from build123d import *


with BuildPart() as part:
    # Sketch1 → Revolve1 (revolve)
    with BuildSketch(Plane.XY, mode=Mode.PRIVATE) as revolve1_sk:
        with BuildLine():
            Line((137.291796068, 0), (141.645898034, 4.868033989))
            ThreePointArc((141.645898034, 4.868033989), (141.910434206, 6.565517768), (140.468847051, 7.5))
            Line((140.468847051, 7.5), (124, 7.5))
            Line((124, 7.5), (124, 5))
            Line((124, 5), (0, 5))
            Line((0, 5), (0, 0))
            Line((0, 0), (124, 0))
            Line((124, 0), (137.291796068, 0))
        make_face()
    revolve1 = revolve(revolve1_sk.sketch.rotate(Axis((0, 0, 0), (1, 0, 0)), 90), axis=Axis((0, 0, 0), (1, 0, 0)))

    # Mirror1: Revolve1 across plane
    add(revolve1.mirror(Plane.ZY))


solid = part.part
Design review of the part built by this model. Coordinates are the model's own, in mm. A direction names the side the tool comes from. Round coordinates to 2 decimals unless told otherwise and drop trailing zeros. Order: outer loops, then holes, each group sorted by start corner. A loop starts at its lowest first (then second) coordinate and runs counter-clockwise, first axis right, second up.
1) Clearance check with flat-ended pins moving along their axes: pin 1 Ø1 at (y, z) = (-1.5, 5.5) entering from +X; pin 2 Ø1.5 at (x, z) = (38.5, -4.5) entering from -Y; pin 3 Ø1 at (x, z) = (75.5, -3) entering from +Y; pin 4 Ø4.5 at (y, z) = (0, 1.5) entering from -X. State where each tip first meets the part, or that it passes through.
The answers:
pin 1: stops at x = 142.05
pin 2: stops at y = -3.31
pin 3: stops at y = 4.33
pin 4: stops at x = -140.65
2) Machinability: for faces 5 (the flat face through (-124, 5, 2)), 6 (the conical face through (-138.05, 0.83, -0.18)), which of the approach directions +Z, -Z, +X, -X, +Y, -Y give a long, thin tool a straight path to every point of the face, cutting with its end or side? Answer none if there is none.
The answers:
face 5: none
face 6: -X
3) Consider section A-A (x = 64). State the section outline as (y, z) points, plus the area to 3 significant figures.
The answers:
outline: circle Ø10 at (0, 0)
area: 78.5 mm2
4) Draft analysis for pull direction X (two halves, no side actions). For faces 1 (the flat face through (124, 5, 2)), 2 (the cylindrical face through (-132.119, -6.324, 4.032)), 3 (the conical face through (138.05, 0.83, -0.18)), 4 (the cylindrical face through (2, 0, -5)), state which applies: released by +X, released by -X, zero draft, split by the parting line, or undercut.
The answers:
face 1: undercut
face 2: zero draft
face 3: released by +X
face 4: undercut
5) For L1, parallel to Y at x = -111.5, z = -1.25; L2, parallel to X at y = -5, z = 2.75; L3, parallel to X at y = 1.5, z = -3.25, list the stretches that pass through material, from the lowest coordinate up.
The answers:
L1: y = -4.84 to 4.84
L2: x = -142.03 to -124, 124 to 142.03
L3: x = -140.49 to 140.49
